```python
from build123d import *

# Parameters (mm, degrees)
SKETCH1_R           = 1.5
SKETCH1_R_2         = 1.236773622
BOSS_EXTRUDE1_DEPTH = 20
SKETCH3_R           = 1.6
CUT_EXTRUDE3_DEPTH  = 29.222331583
CUT_EXTRUDE4_DEPTH  = 14
CUT_EXTRUDE5_START  = -4
CUT_EXTRUDE5_DEPTH  = 25.222331583
SKETCH6_W           = 8.5
SKETCH6_H           = 9
SKETCH6_W_2         = 10
SKETCH6_H_2         = 10.541154273
CUT_EXTRUDE6_DEPTH  = 12.5
CHAMFER2_SIZE       = 2.5
CUT_EXTRUDE7_DEPTH  = 4.5
SKETCH8_R           = 1.55
CUT_EXTRUDE8_DEPTH  = 28.427176304
FILLET1_R           = 4
CHAMFER4_SIZE       = 1.8


with BuildPart() as part:
    # Sketch1 → Boss-Extrude1 (new body)
    with BuildSketch(Plane.XY):
        with BuildLine():
            Line((11, 12.5), (-2.4490752, 3.775186176))
            ThreePointArc((-2.4490752, 3.775186176), (-4.471750095, 0.503439255), (-3.227167472, -3.136142553))
            Line((-3.227167472, -3.136142553), (-1.901778748, -4.5))
            Line((-1.901778748, -4.5), (15, -4.5))
            ThreePointArc((15, -4.5), (19.5, 0), (15, 4.5))
            Line((15, 4.5), (11, 4.5))
            Line((11, 4.5), (11, 12.5))
        make_face()
        Circle(SKETCH1_R, mode=Mode.SUBTRACT)
        with Locations((15, 0)):
            Circle(SKETCH1_R_2, mode=Mode.SUBTRACT)
    extrude(amount=BOSS_EXTRUDE1_DEPTH)

    # Sketch3 → Cut-Extrude3 (cut, through all)
    with BuildSketch(Plane(origin=(11, 0, 0), x_dir=(0, 0, -1), z_dir=(1, 0, 0))):
        with Locations(Location((-18, 7.6, 0), (0, 0, 90))):
            Circle(SKETCH3_R)
    extrude(amount=-CUT_EXTRUDE3_DEPTH, mode=Mode.SUBTRACT)

    # Sketch4 → Cut-Extrude4 (cut)
    with BuildSketch(Plane(origin=(0, 0, 0), x_dir=(-1, 0, 0), z_dir=(0, 0, -1))):
        Polygon((1.58771324, 2.75), (1.58771324, 5.862379977), (6.597571209, 5.862379977), (6.597571209, -6.099785374), (1.58771324, -6.099785374), (1.58771324, -2.75), (-1.58771324, -2.75), (-3.175426481, 0), (-1.58771324, 2.75), align=None)
    extrude(amount=-CUT_EXTRUDE4_DEPTH, mode=Mode.SUBTRACT)

    # Sketch5 → Cut-Extrude5 (cut, through all)
    with BuildSketch(Plane(origin=(11, 0, 0), x_dir=(0, 0, -1), z_dir=(1, 0, 0)).offset(CUT_EXTRUDE5_START)):
        Polygon((-15.3, 6.041154273), (0, 6.041154273), (0, 11.349742261), (-20, 11.872391992), (-20, 5.637009085), (-18, 4.482308546), align=None)
    extrude(amount=-CUT_EXTRUDE5_DEPTH, mode=Mode.SUBTRACT)

    # Sketch6 → Cut-Extrude6 (cut)
    with BuildSketch(Plane(origin=(0, 0, 0), x_dir=(-1, 0, 0), z_dir=(0, 0, -1))):
        with Locations((-15.25, 0)):
            Rectangle(SKETCH6_W, SKETCH6_H)
        with Locations((-0.5, 0.770577137)):
            Rectangle(SKETCH6_W_2, SKETCH6_H_2)
    extrude(amount=-CUT_EXTRUDE6_DEPTH, mode=Mode.SUBTRACT)

    # Chamfer2
    # the kernel refuses this chamfer: 2.5 mm, written as the material it takes off along each edge
    with BuildSketch(Plane(origin=(-1.58771324, -10.92920747, 12.5), x_dir=(-0.027495876610586403, 0, 0.9996219169112968), z_dir=(0, 1, 0))) as chamfer2_piece_1_section:
        Polygon((CHAMFER2_SIZE * 0.999621916911, CHAMFER2_SIZE * 0.0274958766106), (-CHAMFER2_SIZE * 0.0274958766106, CHAMFER2_SIZE * 0.999621916911), (0, 0), align=None)
    chamfer2_piece_1 = extrude(amount=14.60841494, mode=Mode.PRIVATE)
    chamfer2_piece_1 = split(chamfer2_piece_1, bisect_by=Plane(origin=(-0.650189591, -3.625, 14), z_dir=(0, 0, -1)), keep=Keep.TOP, mode=Mode.PRIVATE)
    add(chamfer2_piece_1, mode=Mode.SUBTRACT)
    with BuildSketch(Plane(origin=(-1.58771324, -3.67920747, 12.5), x_dir=(-0.027495876610586403, 0, 0.9996219169112968), z_dir=(0, 1, 0))) as chamfer2_piece_2_section:
        Polygon((CHAMFER2_SIZE * 0.999621916911, CHAMFER2_SIZE * 0.0274958766106), (-CHAMFER2_SIZE * 0.0274958766106, CHAMFER2_SIZE * 0.999621916911), (0, 0), align=None)
    chamfer2_piece_2 = extrude(amount=14.442392157, mode=Mode.PRIVATE)
    chamfer2_piece_2 = split(chamfer2_piece_2, bisect_by=Plane(origin=(-0.650189591, 3.541988609, 14), z_dir=(0, 0, -1)), keep=Keep.TOP, mode=Mode.PRIVATE)
    add(chamfer2_piece_2, mode=Mode.SUBTRACT)

    # Sketch7 → Cut-Extrude7 (cut)
    with BuildSketch(Plane(origin=(0, 0, 12.5), x_dir=(-1, 0, 0), z_dir=(0, 0, -1))):
        Polygon((-12.2, -1.616580754), (-12.2, 1.616580754), (-15, 3.233161507), (-17.8, 1.616580754), (-17.8, -1.616580754), (-15, -3.233161507), align=None)
    extrude(amount=-CUT_EXTRUDE7_DEPTH, mode=Mode.SUBTRACT)

    # Sketch8 → Cut-Extrude8 (cut, through all)
    with BuildSketch(Plane.ZY.offset(-5.5)):
        with Locations(Location((4, 0, 0), (0, 0, 270))):
            Circle(SKETCH8_R)
        with BuildLine():
            Line((12.5, 12.5), (0, 12.5))
            Line((0, 12.5), (0, 0))
            ThreePointArc((0, 0), (3.661165235, 8.838834765), (12.5, 12.5))
        make_face()
    extrude(amount=-CUT_EXTRUDE8_DEPTH, mode=Mode.SUBTRACT)

    # Fillet1
    fillet1_edges = [part.edges().sort_by_distance(p)[0] for p in [
        (8.25, -4.5, 0),
    ]]
    fillet(fillet1_edges, radius=FILLET1_R)

    # Chamfer4
    chamfer4_edges = [part.edges().sort_by_distance(p)[0] for p in [
        (5.5, 1.55, 4),
    ]]
    chamfer(chamfer4_edges, length=CHAMFER4_SIZE)


solid = part.part
```
The model under review builds one solid part; all positions refer to its coordinate system, in mm. A direction names the side the tool comes from. Round coordinates to 2 decimals unless told otherwise and drop trailing zeros. Loops run counter-clockwise (first coordinate to the right, second up) from the corner with the lowest first, then second, coordinate; pieces in that order, holes last. Notation, with made-up numbers: (43.25, 44.25) - (91.25, 44.25) arc R27 cw to (91.25, 72.25) - close; hole circle Ø3 at (58, 64.25). An arc over 180 degrees is marked (long way). Use a Markdown table: item, result. Add a question column.
Q1. Add section A-A (x = 0). State the section outline as (y, z) points, plus the area to 3 significant figures.
Q2. The part is to be moulded in two halves that separate along Y. For faces 4 (the face through (-1.5, 0.07, 16.96)), 5 (the face through (4, 1, 12.5)), 6 (the face through (-2.57, -3.81, 16.96)), say which applies: pulls with the +Y half, pulls with the -Y half, needs draft (parallel to the pull), parting line crosses it, or undercut.
Q3. For probe 1 along X at (y, z) = (0, 16.3); probe 2 along X at (y, z) = (0, 18.8); probe 3 along X at (y, z) = (4.25, 2.25), list the stretches that pass through material, from the lowest coordinate up.
Q4. Add section C-C (x = 3.5). State the section outline as (y, z) points, plus the area to 3 significant figures.
Q5. Insertion check: pin 1 Ø4 at (y, z) = (0, 4) entering from +X; pin 2 Ø3 at (y, z) = (-1, 8.5) entering from -X; pin 3 Ø6.5 at (x, z) = (3.5, 8) entering from +Y. Each pin has a flat end and moves straight along its axis. Give the tip position at first contact, or say it passes through.
Q6. Add section D-D (y = 9.5). State the section outline as (x, z) points.
Q7. Machinability: for faces 1 (the face through (1, 2.75, 13)), 2 (the face through (3.81, 5.25, 16.67)), 3 (the face through (15, -1.4, 17)), which of the approach directions +Z, -Z, +X, -X, +Y, -Y give a long, thin tool a straight path to every point of the face, cutting with its end or side? Answer none if there is none.
Q8. Add section B-B (y = 7.6). State the section outline as (x, z) points, plus the area to 3 significant figures.
Worked answers:
| question | item | result |
|---|---|---|
| 1 | outline | (-4.5, 13.41) - (-2.75, 13.41) - (-2.75, 14) - (-1.5, 14) - (-1.5, 20) - (-4.5, 20) - close; (1.5, 14) - (2.75, 14) - (2.75, 13.41) - (5.36, 13.41) - (5.36, 16.47) - (4.48, 18) - (5.36, 19.53) - (5.36, 20) - (1.5, 20) - close |
| 1 | area | 42.4 mm² |
| 2 | face 4 | undercut |
| 2 | face 5 | needs draft |
| 2 | face 6 | pulls with the -Y half |
| 3 | probe 1 | -4.5 to -1.5, 1.5 to 12.2, 17.8 to 19.5 |
| 3 | probe 2 | -4.5 to -1.5, 1.5 to 13.76, 16.24 to 19.5 |
| 3 | probe 3 | 5.5 to 11 |
| 4 | outline | (-4.5, 12.5) - (6.04, 12.5) - (6.04, 15.3) - (4.48, 18) - (5.64, 20) - (-4.5, 20) - close |
| 4 | area | 75.0 mm² |
| 5 | pin 1 | x = 11 |
| 5 | pin 2 | x = 5.5 |
| 5 | pin 3 | y = 6.04 |
| 6 | outline | (7, 4.38) - (11, 4.38) - (11, 20) - (7, 20) - close |
| 7 | face 1 | -Z, -X |
| 7 | face 2 | -X, +Y |
| 7 | face 3 | -Z |
| 8 | outline | (7, 2.58) - (11, 2.58) - (11, 16.4) - (7, 16.4) - close; (7, 19.6) - (11, 19.6) - (11, 20) - (7, 20) - close |
| 8 | area | 56.9 mm² |
